Work out the finished part from the listing and answer in its coordinate system (mm). Face numbers are marked on the shaded views. A direction names the side the tool comes from. Give positions to 0.01 mm unless a question says otherwise; leave off trailing zeros. Write each loop counter-clockwise with the first axis right and the second up, starting at its lowest first coordinate (ties: lowest second). Pieces come first, ordered by that corner, then holes. Notation, with made-up numbers: (-2.75, 87) -> (5.25, 87) arc R17 ccw to (5.25, 95) -> close; hole circle Ø1 at (-1.75, 62). An arc over 180 degrees is marked (long way). Use a Markdown table: item, result. Add a question column.
Q1. Section A-A, the plane z = 6 is taken. Give the vertices of the cut face in (x, y).
Q2. For a pull along X with two mould halves and no side action, classify the marked faces 1, 2 and 3 as pulls with the +X half, pulls with the -X half, needs draft (parallel to the pull), parting line crosses it, or undercut.
Q3. Section B-B, the plane y = -4 is taken. Give the vertices of the cut face in (x, z), plus the area to 3 significant figures.
Q4. Each of these flat-tipped pins is pushed along its axis until it touches: pin 1 Ø6 at (x, z) = (27.5, 13) entering from +Y; pin 2 Ø6 at (y, z) = (1.45, 6) entering from +X; pin 3 Ø3.5 at (y, z) = (1.45, 19) entering from -X; pin 4 Ø4.5 at (y, z) = (1.45, 19) entering from -X. Where does it stop, or does it pass through?
Q5. For the marked faces 4 and 5, determine the directions among +Z, -Z, +X, -X, +Y, -Y from which every point of the face is accessible in a straight line to the end or side of a thin tool.
Q6. Section C-C, the plane z = 13 is taken. Give the vertices of the cut face in (x, y).
Q7. Consider line 1 (X direction, y = 0.5, z = 15.5); line 2 (Y direction, x = -23.85, z = 19); line 3 (Y direction, x = -21, z = 20). Determine where each line is inside the solid, lowest interval first.
Q8. Section D-D, the plane x = 3 is taken. Give the vertices of the cut face in (y, z).
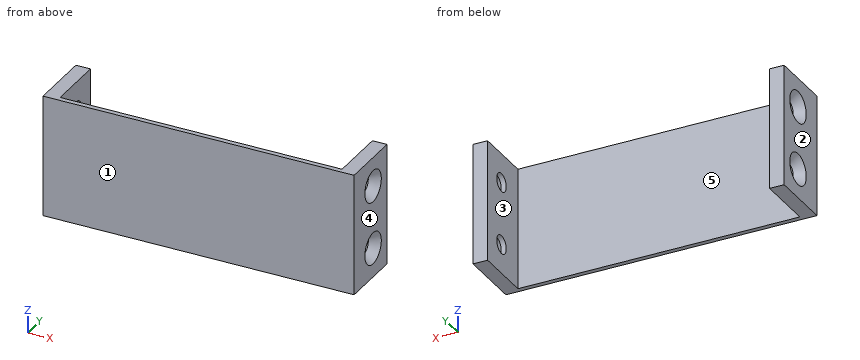
from build123d import *

# Parameters (mm, degrees)
F1_DEPTH       = 25
F4_D           = 3.75
F4_CSINK_D     = 6.5
F4_CSINK_ANGLE = 70
F5_D           = 3.75
F5_CSINK_D     = 6.5
F5_CSINK_ANGLE = 70


with BuildPart() as f1:
    # F0 (on Top) → F1 (new body)
    with BuildSketch(Plane.XY):
        Polygon((-23.20677, 6.948909), (-26.20677, 6.948909), (-26.20677, -6.051091), (37.79323, -6.051091), (37.79323, 6.948909), (34.79323, 6.948909), (34.79323, -5.051091), (-23.20677, -5.051091), align=None)
    extrude(amount=F1_DEPTH)

    # F4 (through all)
    with Locations(Plane(origin=(-26.20677, 0, 0), x_dir=(0, -1, 0), z_dir=(-1, 0, 0))):
        with Locations((-1.448909, 6), (-1.448909, 19)):
            CounterSinkHole(F4_D / 2, F4_CSINK_D / 2, counter_sink_angle=F4_CSINK_ANGLE)

    # F5 (through all)
    with Locations(Plane.YZ.offset(37.79323)):
        with Locations((1.448909, 19), (1.448909, 6)):
            CounterSinkHole(F5_D / 2, F5_CSINK_D / 2, counter_sink_angle=F5_CSINK_ANGLE)


solid = f1.part
Result set:
| question | item | result |
|---|---|---|
| 1 | outline | (-26.21, -6.05) -> (37.79, -6.05) -> (37.79, -1.8) -> (35.83, -0.43) -> (34.79, -0.43) -> (34.79, -5.05) -> (-23.21, -5.05) -> (-23.21, -0.43) -> (-24.24, -0.43) -> (-26.21, -1.8) -> close; (-26.21, 4.7) -> (-24.24, 3.32) -> (-23.21, 3.32) -> (-23.21, 6.95) -> (-26.21, 6.95) -> close; (34.79, 3.32) -> (35.83, 3.32) -> (37.79, 4.7) -> (37.79, 6.95) -> (34.79, 6.95) -> close |
| 2 | face 1 | needs draft |
| 2 | face 2 | pulls with the -X half |
| 2 | face 3 | undercut |
| 3 | outline | (-26.21, 0) -> (-23.21, 0) -> (-23.21, 25) -> (-26.21, 25) -> close; (34.79, 0) -> (37.79, 0) -> (37.79, 25) -> (34.79, 25) -> close |
| 3 | area | 150 mm2 |
| 4 | pin 1 | stops at y = -5.05 |
| 4 | pin 2 | stops at x = 37.44 |
| 4 | pin 3 | passes through |
| 4 | pin 4 | stops at x = -24.78 |
| 5 | face 4 | +Z, -Z, +X, +Y, -Y |
| 5 | face 5 | +Z, -Z, +Y |
| 6 | outline | (-26.21, -6.05) -> (37.79, -6.05) -> (37.79, 6.95) -> (34.79, 6.95) -> (34.79, -5.05) -> (-23.21, -5.05) -> (-23.21, 6.95) -> (-26.21, 6.95) -> close |
| 7 | line 1 | x = -26.21 to -23.21, 34.79 to 37.79 |
| 7 | line 2 | y = -6.05 to -0.43, 3.32 to 6.95 |
| 7 | line 3 | y = -6.05 to -5.05 |
| 8 | outline | (-6.05, 0) -> (-5.05, 0) -> (-5.05, 25) -> (-6.05, 25) -> close |
